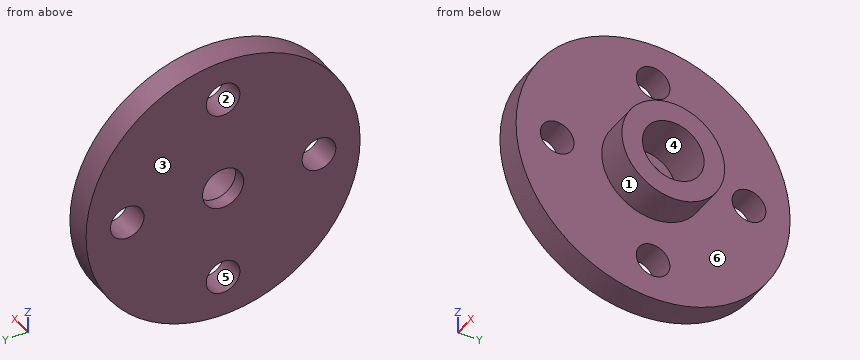
Autodesk Inventor part; units mm, degrees
ref_plane "YZ Plane" through (0, 0, 0) normal (1, 0, 0) x (0, 1, 0)
ref_plane "XZ Plane" through (0, 0, 0) normal (0, 1, 0) x (-1, 0, 0)
ref_plane "XY Plane" through (0, 0, 0) normal (0, 0, 1) x (1, 0, 0)
sketch "Skizze1" plane through (0, 0, 0) normal (0, 0, 1) x (1, 0, 0)
  line L0 (0, 0) -> (4.5, 0)
  line L1 (0, 1.5) -> (1, 1.5)
  line L2 (1, 1.5) -> (1, 2.25)
  line L3 (1, 2.25) -> (4.5, 2.25)
  line L4 (4.5, 2.25) -> (4.5, 3.75)
  line L5 (4.5, 3.75) -> (2, 3.75)
  line L6 (2, 3.75) -> (2, 10)
  line L7 (2, 10) -> (0, 10)
  line L8 (0, 10) -> (0, 1.5)
  point P0 (0.5, 1.5)
  dimension "d0" = 4.5
  dimension "d1" = 3
  dimension "d2" = 1
  dimension "d3" = 7.5
  dimension "d4" = 4.5
  dimension "d5" = 2
  dimension "d6" = 20
revolve "Umdrehung1" add sketch "Skizze1" angle 360 about axis through (0, 0, 0) along (1, 0, 0)
sketch "Skizze2" plane through (2, 0, 0) normal (1, 0, 0) x (0, 0, -1)
  point P0 (0, 0)
  point P1 (0, 7)
  dimension "d8" = 7
hole "Bohrung1" at (2, 7, 0) direction (-1, 0, 0) diameter 2.459 end through all
pattern_circular "Runde Anordnung1" count 4 over 360 about axis through (2.75, 0, 0) along (1, 0, 0) of "Bohrung1"
properties part number "Motor Adapter"
Here's how the part is built. I have some questions about the finished solid (model axes, mm). Face numbers are marked on the shaded views. A direction names the side the tool comes from. Coordinates: 2 decimals unless noted, no trailing zeros. Loops run counter-clockwise (first coordinate to the right, second up) from the corner with the lowest first, then second, coordinate; pieces in that order, holes last. Notation, with made-up numbers: (42.5, -10.5) - (95.5, -10.5) arc R4 cw to (95.5, -6.5) - close; hole circle Ø7 at (-22.75, -22.5). An arc over 180 degrees is marked (long way). Return JSON: item names as keys, results as strings. Group by question number.
Item 1: We'd pull the mould along Z, two halves only. Please class the marked faces 1, 2, 3 and 4: +Z half, -Z half, draft (parallel to the pull), parting line (faces both ways), or undercut.
Item 2: Will these pins go through, and if not, where does the flat tip stop? P1, Ø1.5, axis at x = 1, z = -8, coming from the +Y side; P2, Ø1.5, axis at y = 8, z = 4, coming from the +X side.
Item 3: I need wall thicknesses on line 1 (Z direction, x = 0.8, y = 0); line 2 (Z direction, x = 1.2, y = 0); line 3 (Z direction, x = 3.4, y = 0). Which ranges of each line are inside material? Lowest first, please. Write a range as from..to.
Item 4: If we section it at C-C on y = 7: Write out the boundary of the cut face in (x, z), and give its area (3 significant figures).
Item 5: If we section it at D-D on x = 0.75: Write out the boundary of the cut face in (y, z), and give its area (3 significant figures).
Item 6: If we section it at A-A on y = 0: Write out the boundary of the cut face in (x, z), and give its area (3 significant figures).
Item 7: If we section it at B-B on z = 0.25: Write out the boundary of the cut face in (x, y).
Item 8: On a 3-axis mill with a long thin cutter (end or side, diameter ignored), from which of +Z, -Z, +X, -X, +Y, -Y can I reach the whole of each face in a straight line? I mean the marked faces 5 and 6. Say none if no direction works.
Calculated:
{
 "1": {"face 1": "parting line", "face 2": "undercut", "face 3": "draft", "face 4": "undercut"},
 "2": {"P1": "stops at y = 6.89", "P2": "stops at x = 2"},
 "3": {"line 1": "z = -10..-8.23, -5.77..-1.5, 1.5..5.77, 8.23..10", "line 2": "z = -10..-8.23, -5.77..-2.25, 2.25..5.77, 8.23..10", "line 3": "z = -3.75..-2.25, 2.25..3.75"},
 "4": {"outline": "(0, -7.14) - (2, -7.14) - (2, -1.23) - (0, -1.23) - close; (0, 1.23) - (2, 1.23) - (2, 7.14) - (0, 7.14) - close", "area": "23.6 mm^2"},
 "5": {"outline": "circle Ø20 at (0, 0); hole circle Ø2.46 at (-7, 0); hole circle Ø3 at (0, 0); hole circle Ø2.46 at (0, -7); hole circle Ø2.46 at (0, 7); hole circle Ø2.46 at (7, 0)", "area": "288 mm^2"},
 "6": {"outline": "(0, -10) - (2, -10) - (2, -8.23) - (0, -8.23) - close; (0, -5.77) - (2, -5.77) - (2, -3.75) - (4.5, -3.75) - (4.5, -2.25) - (1, -2.25) - (1, -1.5) - (0, -1.5) - close; (0, 1.5) - (1, 1.5) - (1, 2.25) - (4.5, 2.25) - (4.5, 3.75) - (2, 3.75) - (2, 5.77) - (0, 5.77) - close; (0, 8.23) - (2, 8.23) - (2, 10) - (0, 10) - close", "area": "30.2 mm^2"},
 "7": {"outline": "(0, -10) - (2, -10) - (2, -8.2) - (0, -8.2) - close; (0, -5.8) - (2, -5.8) - (2, -3.74) - (4.5, -3.74) - (4.5, -2.24) - (1, -2.24) - (1, -1.48) - (0, -1.48) - close; (0, 1.48) - (1, 1.48) - (1, 2.24) - (4.5, 2.24) - (4.5, 3.74) - (2, 3.74) - (2, 5.8) - (0, 5.8) - close; (0, 8.2) - (2, 8.2) - (2, 10) - (0, 10) - close"},
 "8": {"face 5": "+X, -X", "face 6": "+X"}
}
